For this review, take the finished solid that the model builds, in its own axes (mm). A direction names the side the tool comes from. Coordinates: 2 decimals unless noted, no trailing zeros. Loops run counter-clockwise (first coordinate to the right, second up) from the corner with the lowest first, then second, coordinate; pieces in that order, holes last.
1. Take a section at A-A, the plane y = 5. State the section outline as (x, z) points.
2. Clearance check with flat-ended pins moving along their axes: P1, Ø0.8, axis at y = -2.5, z = 2.5, coming from the +X side; P2, Ø6, axis at x = 2, y = -4.5, coming from the -Z side; P3, Ø10, axis at x = -10.5, y = 0, coming from the +Z side; P4, Ø1.5, axis at x = -21, y = -7, coming from the +Z side. State where each tip first meets the part, or that it passes through.
3. Take a section at D-D, the plane y = -9.5. State the section outline as (x, z) points.
4. To check wall thickness, follow probe 1 along X at (y, z) = (3, 2.75); probe 2 along X at (y, z) = (-4.5, 0.5); probe 3 along X at (y, z) = (-2, 2.25). State the ranges of each line that lie inside material, in increasing order.
5. Take a section at C-C, the plane z = 1. State the section outline as (x, y) points, then the cut area to 3 significant figures.
6. Take a section at B-B, the plane x = -3. State the section outline as (y, z) points.
7. Machinability: for faces 5 (the face through (-22.8, -4.613, 3.8)), 6 (the face through (15.3, 0.387, 3.7)), 7 (the face through (-22.7, 3.387, 3.8)), which of the approach directions +Z, -Z, +X, -X, +Y, -Y give a long, thin tool a straight path to every point of the face, cutting with its end or side? Answer none if there is none.
8. Mouldability with a two-part tool opening along Y and no side actions: class faces 1 (the face through (-22.8, -4.113, 3.8)), 2 (the face through (12.8, 1.887, 2.5)), 3 (the face through (15.3, -1.613, 3.7)), 4 (the face through (12.8, -3.113, 2.5)) as pulls with the +Y half, pulls with the -Y half, needs draft (parallel to the pull), parting line crosses it, or undercut.
```python
from build123d import *

# Parameters (mm, degrees)
SKETCH1_W           = 40
SKETCH1_H           = 20
BOSS_EXTRUDE1_DEPTH = 2
SKETCH2_W           = 3
SKETCH2_H           = 10
SKETCH2_H_2         = 5
BOSS_EXTRUDE2_DEPTH = 1
SKETCH3_W           = 0.5
SKETCH3_H           = 0.5
BOSS_EXTRUDE3_DEPTH = 1
SKETCH5_W           = 0.415981526
SKETCH5_H           = 0.5
BOSS_EXTRUDE4_DEPTH = 5
FILLET1_R           = 0.2
SKETCH7_W           = 0.477868842
SKETCH7_H           = 0.5
BOSS_EXTRUDE5_DEPTH = 5
FILLET3_R           = 0.2
SKETCH8_W           = 5.346247603
SKETCH8_H           = 4.799297503
BOSS_EXTRUDE6_DEPTH = 5
BOSS_EXTRUDE8_DEPTH = 1
CUT_EXTRUDE1_REACH  = 30.088
SKETCH10_R          = 2.349261849
SKETCH13_R          = 3.48485592
BOSS_EXTRUDE9_DEPTH = 1
CUT_EXTRUDE2_REACH  = 30.088
SKETCH14_R          = 2.382418239
FILLET5_R           = 0.2


with BuildPart() as part:
    # Sketch1 → Boss-Extrude1 (new body)
    with BuildSketch(Plane.XY):
        with Locations((-3.443579767, -0.612840467)):
            Rectangle(SKETCH1_W, SKETCH1_H)
    extrude(amount=BOSS_EXTRUDE1_DEPTH)

    # Sketch2 → Boss-Extrude2 (add)
    with BuildSketch(Plane.XY.offset(2)):
        with Locations((-20.270719319, -0.612840467)):
            Rectangle(SKETCH2_W, SKETCH2_H)
        with Locations((12.857244344, -0.612840467)):
            Rectangle(SKETCH2_W, SKETCH2_H_2)
    extrude(amount=BOSS_EXTRUDE2_DEPTH)

    # Sketch3 → Boss-Extrude3 (add)
    with BuildSketch(Plane.XY.offset(3)):
        with Locations((-20.270719319, 3.137159533)):
            Rectangle(SKETCH3_W, SKETCH3_H)
        with Locations((-20.270719319, 0.637159533)):
            Rectangle(SKETCH3_W, SKETCH3_H)
        with Locations((-20.270719319, -1.862840467)):
            Rectangle(SKETCH3_W, SKETCH3_H)
        with Locations((-20.270719319, -4.362840467)):
            Rectangle(SKETCH3_W, SKETCH3_H)
        with Locations((12.857244344, -1.862840467)):
            Rectangle(SKETCH3_W, SKETCH3_H)
        with Locations((12.857244344, 0.637159533)):
            Rectangle(SKETCH3_W, SKETCH3_H)
    extrude(amount=BOSS_EXTRUDE3_DEPTH)

    # Sketch5 → Boss-Extrude4 (add)
    with BuildSketch(Plane.ZY.offset(20.520719319)):
        with Locations((3.792009237, 3.137159533)):
            Rectangle(SKETCH5_W, SKETCH5_H)
        with Locations((3.792009237, 0.637159533)):
            Rectangle(SKETCH5_W, SKETCH5_H)
        with Locations((3.792009237, -1.862840467)):
            Rectangle(SKETCH5_W, SKETCH5_H)
        with Locations((3.792009237, -4.362840467)):
            Rectangle(SKETCH5_W, SKETCH5_H)
    extrude(amount=BOSS_EXTRUDE4_DEPTH)

    # Fillet1
    fillet1_edges = [part.edges().sort_by_distance(p)[0] for p in [
        (-20.020719319, 3.137159533, 4),
        (-20.020719319, 0.637159533, 4),
        (-20.020719319, -1.862840467, 4),
        (-20.020719319, -4.362840467, 4),
    ]]
    fillet(fillet1_edges, radius=FILLET1_R)

    # Sketch7 → Boss-Extrude5 (add)
    with BuildSketch(Plane(origin=(13.107244344, 0, 0), x_dir=(0, 0, -1), z_dir=(1, 0, 0))):
        with Locations((-3.761065579, -1.862840467)):
            Rectangle(SKETCH7_W, SKETCH7_H)
        with Locations((-3.761065579, 0.637159533)):
            Rectangle(SKETCH7_W, SKETCH7_H)
    extrude(amount=BOSS_EXTRUDE5_DEPTH)

    # Fillet3
    fillet3_edges = [part.edges().sort_by_distance(p)[0] for p in [
        (12.607244344, -1.862840467, 4),
        (12.607244344, 0.637159533, 4),
    ]]
    fillet(fillet3_edges, radius=FILLET3_R)

    # Sketch8 → Boss-Extrude6 (add)
    with BuildSketch(Plane.XY.offset(2)):
        with Locations((-2.673123802, 4.786787988)):
            Rectangle(SKETCH8_W, SKETCH8_H)
    extrude(amount=BOSS_EXTRUDE6_DEPTH)

    # Sketch9 → Boss-Extrude8 (add)
    with BuildSketch(Plane.XY.offset(2)):
        Polygon((0.091656416, -4.824510849), (-0.615226542, -4.824510849), (-0.615226542, -4.128822948), (0.091656416, -4.128822948), (0.091656416, -3.824510849), (-0.615226542, -3.824510849), (-0.615226542, -3.128822948), (0.091656416, -3.128822948), (0.091656416, -2.824510849), (-0.615226542, -2.824510849), (-0.615226542, -2.128822948), (0.091656416, -2.128822948), (0.091656416, -1.902319725), (0.43302666, -1.902319725), (0.43302666, -1.202319725), (1.13302666, -1.202319725), (1.13302666, -1.902319725), (1.43302666, -1.902319725), (1.43302666, -1.202319725), (2.13302666, -1.202319725), (2.13302666, -1.902319725), (2.43302666, -1.902319725), (2.43302666, -1.202319725), (3.13302666, -1.202319725), (3.13302666, -1.902319725), (3.43302666, -1.902319725), (3.43302666, -1.202319725), (4.13302666, -1.202319725), (4.13302666, -1.902319725), (4.266316816, -1.902319725), (4.266316816, -2.154701216), (4.966316816, -2.154701216), (4.966316816, -2.854701216), (4.266316816, -2.854701216), (4.266316816, -3.154701216), (4.966316816, -3.154701216), (4.966316816, -3.854701216), (4.266316816, -3.854701216), (4.266316816, -4.154701216), (4.966316816, -4.154701216), (4.966316816, -4.854701216), (4.266316816, -4.854701216), (4.266316816, -5.154701216), (4.966316816, -5.154701216), (4.966316816, -5.854701216), (4.266316816, -5.854701216), (4.266316816, -6.07698014), (4.077584514, -6.07698014), (4.077584514, -6.77698014), (3.377584514, -6.77698014), (3.377584514, -6.07698014), (3.077584514, -6.07698014), (3.077584514, -6.77698014), (2.377584514, -6.77698014), (2.377584514, -6.07698014), (2.077584514, -6.07698014), (2.077584514, -6.77698014), (1.377584514, -6.77698014), (1.377584514, -6.07698014), (1.077584514, -6.07698014), (1.077584514, -6.77698014), (0.377584514, -6.77698014), (0.377584514, -6.07698014), (0.091656416, -6.07698014), (0.091656416, -5.824510849), (-0.615226542, -5.824510849), (-0.615226542, -5.128822948), (0.091656416, -5.128822948), align=None)
    extrude(amount=BOSS_EXTRUDE8_DEPTH)

    # Sketch10 → Cut-Extrude1 (cut, up to next)
    with BuildSketch(Plane.XY.offset(2), mode=Mode.PRIVATE) as cut_extrude1_sk1:
        with Locations((-11.713689096, -4.527627409)):
            Circle(SKETCH10_R)
    cut_extrude1_tool1 = extrude(cut_extrude1_sk1.sketch, amount=-CUT_EXTRUDE1_REACH, mode=Mode.PRIVATE) & part.part
    add(cut_extrude1_tool1.solids().sort_by_distance((-11.713689, -4.527627, 2))[0], mode=Mode.SUBTRACT)

    # Sketch13 → Boss-Extrude9 (add)
    with BuildSketch(Plane.XY.offset(2)):
        with Locations((-11.713689096, -4.527627409)):
            Circle(SKETCH13_R)
    extrude(amount=BOSS_EXTRUDE9_DEPTH)

    # Sketch14 → Cut-Extrude2 (cut, up to next)
    with BuildSketch(Plane(origin=(0, 0, 2), x_dir=(-1, 0, 0), z_dir=(0, 0, -1)), mode=Mode.PRIVATE) as cut_extrude2_sk1:
        with Locations((11.713689096, -4.527627409)):
            Circle(SKETCH14_R)
    cut_extrude2_tool1 = extrude(cut_extrude2_sk1.sketch, amount=-CUT_EXTRUDE2_REACH, mode=Mode.PRIVATE) & part.part
    add(cut_extrude2_tool1.solids().sort_by_distance((-11.713689, -4.527627, 2))[0], mode=Mode.SUBTRACT)

    # Fillet5
    fillet5_edges = [part.edges().sort_by_distance(p)[0] for p in [
        (-15.198545015, -4.527627409, 3),
        (-9.331270856, -4.527627409, 3),
    ]]
    fillet(fillet5_edges, radius=FILLET5_R)


solid = part.part
```
Results list:
1. outline: (-23.44, 0) - (16.56, 0) - (16.56, 2) - (0, 2) - (0, 7) - (-5.35, 7) - (-5.35, 2) - (-23.44, 2) - close
2. P1: stops at x = 14.36
2. P2: stops at z = 0
2. P3: stops at z = 3
2. P4: stops at z = 2
3. outline: (-23.44, 0) - (16.56, 0) - (16.56, 2) - (-23.44, 2) - close
4. probe 1: x = -21.77 to -18.77, -5.35 to 0
4. probe 2: x = -23.44 to -14.06, -9.36 to 16.56
4. probe 3: x = -21.77 to -18.77, -14.11 to -9.31, 0.09 to 4.27, 11.36 to 14.36
5. outline: (-23.44, -10.61) - (16.56, -10.61) - (16.56, 9.39) - (-23.44, 9.39) - close; hole circle Ø4.7 at (-11.71, -4.53)
5. area: 783 mm2
6. outline: (-10.61, 0) - (9.39, 0) - (9.39, 2) - (7.19, 2) - (7.19, 7) - (2.39, 7) - (2.39, 2) - (-10.61, 2) - close
7. face 5: +Z, +X, -X, -Y
7. face 6: +Z, +X, -X
7. face 7: +Z, -X, +Y
8. face 1: undercut
8. face 2: pulls with the +Y half
8. face 3: undercut
8. face 4: pulls with the -Y half
